from build123d import *

# Parameters (mm, degrees)
F1_DEPTH  = 55
F3_R      = 4
F4_DEPTH  = 50
F5_R      = 4
F6_DEPTH  = 100
F8_R      = 3.3
F9_DEPTH  = 25
F10_R     = 3.3
F11_DEPTH = 25


with BuildPart() as f1:
    # F0 (on Top) → F1 (new body)
    with BuildSketch(Plane.XY):
        with BuildLine():
            Line((20.5, 0), (0, 0))
            Line((0, 0), (0, -19.5))
            Line((0, -19.5), (-25.5, -19.5))
            Line((-25.5, -19.5), (-25.5, -31.5))
            Line((-25.5, -31.5), (-9.9330343737, -31.5))
            ThreePointArc((-9.9330343737, -31.5), (5, -32.5), (-9.9330343737, -33.5))
            Line((-9.9330343737, -33.5), (-25.5, -33.5))
            Line((-25.5, -33.5), (-25.5, -45.5))
            Line((-25.5, -45.5), (0, -45.5))
            Line((0, -45.5), (0, -65))
            Line((0, -65), (20.5, -65))
            Line((20.5, -65), (20.5, 0))
        make_face()
    extrude(amount=F1_DEPTH)

    # F3 (on offset) → F4 (cut, symmetric)
    with BuildSketch(Plane.XZ.offset(45.5)):
        with Locations((-16.5, 10)):
            Circle(F3_R)
    extrude(amount=F4_DEPTH, both=True, mode=Mode.SUBTRACT)

    # F5 (on offset) → F6 (cut)
    with BuildSketch(Plane.XZ.offset(45.5)):
        with Locations((-16.5, 45)):
            Circle(F5_R)
    extrude(amount=-F6_DEPTH, mode=Mode.SUBTRACT)

    # F8 (on offset) → F9 (cut)
    with BuildSketch(Plane(origin=(0, 0, 0), x_dir=(0, -1, 0), z_dir=(-1, 0, 0))):
        with Locations((9.25, 45)):
            Circle(F8_R)
        with Locations((9.25, 10)):
            Circle(F8_R)
    extrude(amount=-F9_DEPTH, mode=Mode.SUBTRACT)

    # F10 (on offset) → F11 (cut)
    with BuildSketch(Plane(origin=(0, 0, 0), x_dir=(0, -1, 0), z_dir=(-1, 0, 0))):
        with Locations((56, 10)):
            Circle(F10_R)
        with Locations((56, 45)):
            Circle(F10_R)
    extrude(amount=-F11_DEPTH, mode=Mode.SUBTRACT)


solid = f1.part
Could you check a few things on this model? Use its own coordinates, in mm. A direction names the side the tool comes from. Give positions to 0.01 mm unless a question says otherwise; leave off trailing zeros. Loops run counter-clockwise (first coordinate to the right, second up) from the corner with the lowest first, then second, coordinate; pieces in that order, holes last. Notation, with made-up numbers: M 28,56.5 L 77,56.5 A23 ccw 77,83.5 Z; hole C 68.5,33 d4. An arc over 180 degrees is marked long. Answer as a JSON object with one key per item and string values.
Q1. For P1, Ø1.5, axis at x = -8.5, z = 26.5, coming from the +Y side; P2, Ø8, axis at y = -57, z = 34, coming from the -X side; P3, Ø10.5, axis at x = -16.5, z = 10, coming from the -Y side, each with a flat end and sliding along its axis, tell me the tip position at first contact or that it passes through.
Values found:
{"P1": "stops at y = -19.5", "P2": "stops at x = 0", "P3": "stops at y = -45.5"}
Q2. Suppose I cut it at B-B, the plane y = -56. List the corners of the cut face in (x, z) for me, plus the area to 3 significant figures.
Values found:
{"outline": "M 0,0 L 20.5,0 L 20.5,6.7 L 0,6.7 Z; M 0,13.3 L 20.5,13.3 L 20.5,41.7 L 0,41.7 Z; M 0,48.3 L 20.5,48.3 L 20.5,55 L 0,55 Z", "area": "857 mm²"}
Q3. Suppose I cut it at D-D, the plane x = -11. List the corners of the cut face in (y, z) for me.
Values found:
{"outline": "M -45.5,0 L -33.5,0 L -33.5,55 L -45.5,55 Z; M -31.5,0 L -19.5,0 L -19.5,55 L -31.5,55 Z"}
Q4. For faces 4 (the flat face through (-18, -33.5, 27)), 5 (the flat face through (-13, -19.5, 27)), 6 (the flat face through (0, -55, 27)), 7 (the cylindrical face through (-20.496, -39.584, 10.176)), which set-ups out of +Z, -Z, +X, -X, +Y, -Y let a thin tool reach every point of the face, with its end or its side?
Values found:
{"face 4": "+Z, -Z, -X", "face 5": "+Z, -Z, -X, +Y", "face 6": "+Z, -Z, -X, -Y", "face 7": "+Y, -Y"}
Q5. If we mould it in two halves opening along X, with no side actions, what happens to faces 1 (the flat face through (-25.5, -25, 27)), 2 (the cylindrical face through (-20.496, -25.584, 10.176)), 3 (the cylindrical face through (10.11, -8.82, 48.27))? For each: pulls with the +X half, pulls with the -X half, needs draft (parallel to the pull), parting line crosses it, or undercut.
Values found:
{"face 1": "pulls with the -X half", "face 2": "undercut", "face 3": "needs draft"}
Q6. Suppose I cut it at A-A, the plane x = -16.5. List the corners of the cut face in (y, z) for me.
Values found:
{"outline": "M -45.5,0 L -33.5,0 L -33.5,6 L -45.5,6 Z; M -45.5,14 L -33.5,14 L -33.5,41 L -45.5,41 Z; M -45.5,49 L -33.5,49 L -33.5,55 L -45.5,55 Z; M -31.5,0 L -19.5,0 L -19.5,6 L -31.5,6 Z; M -31.5,14 L -19.5,14 L -19.5,41 L -31.5,41 Z; M -31.5,49 L -19.5,49 L -19.5,55 L -31.5,55 Z"}
Q7. If I drill on probe 1 along Z at (x, y) = (7, -9); probe 2 along Z at (x, y) = (-16.5, -42.5); probe 3 along Y at (x, z) = (-23, 2), over which ranges is the centre line in solid material (lowest first)? Write a range as [from, to].
Values found:
{"probe 1": "z = [0, 6.71], [13.29, 41.71], [48.29, 55]", "probe 2": "z = [0, 6], [14, 41], [49, 55]", "probe 3": "y = [-45.5, -33.5], [-31.5, -19.5]"}
Q8. Suppose I cut it at C-C, the plane z = 45. List the corners of the cut face in (x, y) for me.
Values found:
{"outline": "M -25.5,-45.5 L -20.5,-45.5 L -20.5,-33.5 L -25.5,-33.5 Z; M -25.5,-31.5 L -20.5,-31.5 L -20.5,-19.5 L -25.5,-19.5 Z; M -12.5,-45.5 L 0,-45.5 L 0,-52.7 L 20.5,-52.7 L 20.5,-12.55 L 0,-12.55 L 0,-19.5 L -12.5,-19.5 L -12.5,-31.5 L -9.93,-31.5 A7.5 cw long -9.93,-33.5 L -12.5,-33.5 Z; M 0,-65 L 20.5,-65 L 20.5,-59.3 L 0,-59.3 Z; M 0,-5.95 L 20.5,-5.95 L 20.5,0 L 0,0 Z"}
